Build history of the part. All positions in model axes, mm. Round coordinates to 2 decimals unless told otherwise and drop trailing zeros. Loops run counter-clockwise (first coordinate to the right, second up) from the corner with the lowest first, then second, coordinate; pieces in that order, holes last. Notation, with made-up numbers: (71, 32) -> (100, 32) arc R30 cw to (100, 62) -> close; hole circle Ø5 at (-23.75, 59.5). An arc over 180 degrees is marked (long way). Put each result on its own line as item: value. Start each with the question number.
Item 1: Cut at D-D, the plane z = -1.45. Count the separate pieces of the cut face and the enclosed holes in it, plus the area to 3 significant figures.
Item 2: Cut at B-B, the plane y = 0. List the corners of the cut face in (x, z) (3 decimals).
Item 3: Drill centre lines: probe 1 along X at (y, z) = (-52.5, -2.7); probe 2 along X at (y, z) = (5, -2.2); probe 3 along X at (y, z) = (39.5, -1.15). Where is each one in solid material? Low to high. Write a range as [from, to].
Item 4: Flat gauge pins, fed straight in: pin 1 Ø1.6 at (x, y) = (61.62, -80.69) entering from -Z; pin 2 Ø2.5 at (x, y) = (75.03, -55.96) entering from -Z (3 decimals). Where does each tip first touch, or does it go through?
Item 5: Cut at C-C, the plane y = 24.5. List the corners of the cut face in (x, z) (3 decimals), plus the area to 3 significant figures.
Item 6: Cut at A-A, the plane x = 0. List the corners of the cut face in (y, z) (3 decimals), plus the area to 3 significant figures.
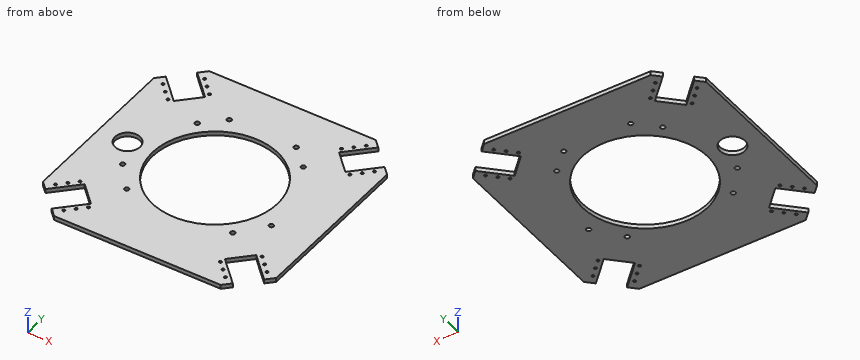
```python
from build123d import *

# Parameters (mm, degrees)
SKETCH1_R          = 9.525
SKETCH1_R_2        = 0.9906
SKETCH1_R_3        = 47.625
EXTRUDE1_DEPTH     = 3.175
SKETCH2_R          = 1.7272
CUT_EXTRUDE1_DEPTH = 3.175
SPLIT1_START       = -3.175
SPLIT1_OUTLINE_R   = 1.7272
SPLIT1_DEPTH       = 3.175


# Read off the part's stored shape, not the designer's step: Split1
with BuildPart() as part:
    # Sketch1 → Extrude1 (new body)
    with BuildSketch(Plane.XY):
        Polygon((-88.9, 63.5), (-83.384204897, 69.015795103), (-65.423692655, 51.055282861), (-51.055282861, 65.423692655), (-69.015795103, 83.384204897), (-63.5, 88.9), (63.5, 88.9), (69.015795103, 83.384204897), (51.055282861, 65.423692655), (65.423692655, 51.055282861), (83.384204897, 69.015795103), (88.9, 63.5), (88.9, -63.5), (83.384204897, -69.015795103), (65.423692655, -51.055282861), (51.055282861, -65.423692655), (69.015795103, -83.384204897), (63.5, -88.9), (-63.5, -88.9), (-69.015795103, -83.384204897), (-51.055282861, -65.423692655), (-65.423692655, -51.055282861), (-83.384204897, -69.015795103), (-88.9, -63.5), align=None)
        with Locations((-66.675, 0)):
            Circle(SKETCH1_R, mode=Mode.SUBTRACT)
        with Locations((-80.690128061, 61.616064059)):
            Circle(SKETCH1_R_2, mode=Mode.SUBTRACT)
        with Locations((-75.032566704, 55.958502703)):
            Circle(SKETCH1_R_2, mode=Mode.SUBTRACT)
        with Locations((-69.375005348, 50.300941347)):
            Circle(SKETCH1_R_2, mode=Mode.SUBTRACT)
        with Locations(Location((-50.300941347, 69.375005348, 0), (0, 0, 180))):
            Circle(SKETCH1_R_2, mode=Mode.SUBTRACT)
        with Locations(Location((-55.958502703, 75.032566704, 0), (0, 0, 180))):
            Circle(SKETCH1_R_2, mode=Mode.SUBTRACT)
        with Locations(Location((-61.616064059, 80.690128061, 0), (0, 0, 180))):
            Circle(SKETCH1_R_2, mode=Mode.SUBTRACT)
        with Locations((50.300941347, 69.375005348)):
            Circle(SKETCH1_R_2, mode=Mode.SUBTRACT)
        with Locations((55.958502703, 75.032566704)):
            Circle(SKETCH1_R_2, mode=Mode.SUBTRACT)
        with Locations((61.616064059, 80.690128061)):
            Circle(SKETCH1_R_2, mode=Mode.SUBTRACT)
        with Locations(Location((69.375005348, 50.300941347, 0), (0, 0, 180))):
            Circle(SKETCH1_R_2, mode=Mode.SUBTRACT)
        with Locations(Location((75.032566704, 55.958502703, 0), (0, 0, 180))):
            Circle(SKETCH1_R_2, mode=Mode.SUBTRACT)
        with Locations(Location((80.690128061, 61.616064059, 0), (0, 0, 180))):
            Circle(SKETCH1_R_2, mode=Mode.SUBTRACT)
        with Locations((80.690128061, -61.616064059)):
            Circle(SKETCH1_R_2, mode=Mode.SUBTRACT)
        with Locations((75.032566704, -55.958502703)):
            Circle(SKETCH1_R_2, mode=Mode.SUBTRACT)
        with Locations((69.375005348, -50.300941347)):
            Circle(SKETCH1_R_2, mode=Mode.SUBTRACT)
        with Locations(Location((61.616064059, -80.690128061, 0), (0, 0, 180))):
            Circle(SKETCH1_R_2, mode=Mode.SUBTRACT)
        with Locations(Location((55.958502703, -75.032566704, 0), (0, 0, 180))):
            Circle(SKETCH1_R_2, mode=Mode.SUBTRACT)
        with Locations(Location((50.300941347, -69.375005348, 0), (0, 0, 180))):
            Circle(SKETCH1_R_2, mode=Mode.SUBTRACT)
        with Locations((-61.616064059, -80.690128061)):
            Circle(SKETCH1_R_2, mode=Mode.SUBTRACT)
        with Locations((-55.958502703, -75.032566704)):
            Circle(SKETCH1_R_2, mode=Mode.SUBTRACT)
        with Locations((-50.300941347, -69.375005348)):
            Circle(SKETCH1_R_2, mode=Mode.SUBTRACT)
        with Locations(Location((-80.690128061, -61.616064059, 0), (0, 0, 180))):
            Circle(SKETCH1_R_2, mode=Mode.SUBTRACT)
        with Locations(Location((-75.032566704, -55.958502703, 0), (0, 0, 180))):
            Circle(SKETCH1_R_2, mode=Mode.SUBTRACT)
        with Locations(Location((-69.375005348, -50.300941347, 0), (0, 0, 180))):
            Circle(SKETCH1_R_2, mode=Mode.SUBTRACT)
        Circle(SKETCH1_R_3, mode=Mode.SUBTRACT)
    extrude(amount=-EXTRUDE1_DEPTH)

    # Sketch2 → Cut-Extrude1 (cut)
    with BuildSketch(Plane(origin=(0, 0, -3.175), x_dir=(-1, 0, 0), z_dir=(0, 0, -1))):
        with Locations((-40.411152545, -40.411152545)):
            Circle(SKETCH2_R)
        with Locations((40.411152545, 40.411152545)):
            Circle(SKETCH2_R)
        with Locations((40.411152545, -40.411152545)):
            Circle(SKETCH2_R)
        with Locations((-40.411152545, 40.411152545)):
            Circle(SKETCH2_R)
    extrude(amount=-CUT_EXTRUDE1_DEPTH, mode=Mode.SUBTRACT)

    # Split1 outline → Split1 (cut)
    with BuildSketch(Plane.XY.offset(SPLIT1_START)):
        with Locations((25.49444664, 54.673017253)):
            Circle(SPLIT1_OUTLINE_R)
        with Locations((-56.686957349, -20.632365146)):
            Circle(SPLIT1_OUTLINE_R)
        with Locations((-25.49444664, 54.673017253)):
            Circle(SPLIT1_OUTLINE_R)
        with Locations((56.686957349, -20.632365146)):
            Circle(SPLIT1_OUTLINE_R)
    extrude(amount=SPLIT1_DEPTH, mode=Mode.SUBTRACT)


solid = part.part
```
Reply:
1. separate pieces: 1
1. enclosed holes: 34
1. area: 20,700 mm^2
2. outline: (-88.9, -3.175) -> (-76.2, -3.175) -> (-76.2, 0) -> (-88.9, 0) -> close; (-57.15, -3.175) -> (-47.625, -3.175) -> (-47.625, 0) -> (-57.15, 0) -> close; (47.625, -3.175) -> (88.9, -3.175) -> (88.9, 0) -> (47.625, 0) -> close
3. probe 1: x = [-88.9, -66.87], [-63.98, 63.98], [66.87, 88.9]
3. probe 2: x = [-88.9, -74.78], [-58.57, -47.36], [47.36, 88.9]
3. probe 3: x = [-88.9, -41.88], [-38.94, -26.61], [26.61, 38.94], [41.88, 88.9]
4. pin 1: passes through
4. pin 2: stops at z = -3.175
5. outline: (-88.9, -3.175) -> (-40.84, -3.175) -> (-40.84, 0) -> (-88.9, 0) -> close; (40.84, -3.175) -> (88.9, -3.175) -> (88.9, 0) -> (40.84, 0) -> close
5. area: 305 mm^2
6. outline: (-88.9, -3.175) -> (-47.625, -3.175) -> (-47.625, 0) -> (-88.9, 0) -> close; (47.625, -3.175) -> (88.9, -3.175) -> (88.9, 0) -> (47.625, 0) -> close
6. area: 262 mm^2
